Here's how the part is built. I have some questions about the finished solid (model axes, mm). Round coordinates to 2 decimals unless told otherwise and drop trailing zeros. Write each loop counter-clockwise with the first axis right and the second up, starting at its lowest first coordinate (ties: lowest second). Pieces come first, ordered by that corner, then holes. Notation, with made-up numbers: (35, 21) - (43, 21) arc R7 cw to (43, 30) - close; hole circle Ø7 at (-20.5, 4). An arc over 180 degrees is marked (long way). Use one line per item in the form item = value. Start each with the question number.
1. I want a section at B-B, the plane y = -19. List the corners of the cut face in (x, z) for me.
2. I want a section at A-A, the plane x = -59. List the corners of the cut face in (y, z) for me.
3. If I drill on line 1 along Y through (x, z) = (-31.5, -9.25); line 2 along Z through (x, y) = (-53, -25.5); line 3 along Y through (x, z) = (-32, 1.25), over which ranges is the centre line in solid material (lowest first)?
4. I want a section at C-C, the plane z = -15.75. List the corners of the cut face in (x, y) for me.
5. Will these pins go through, and if not, where does the flat tip stop? pin 1 (12 mm diameter, centred on x = -41.5, z = -4.5, fed in from +Y); pin 2 (3 mm diameter, centred on y = -25, z = -6.5, fed in from +X); pin 3 (1.8 mm diameter, centred on y = -25.5, z = -14, fed in from -X); pin 4 (6 mm diameter, centred on x = -67, y = -10, fed in from -Z).
```python
from build123d import *

# Parameters (mm, degrees)
CROQUIS1_W              = 50
CROQUIS1_H              = 50
CROQUIS1_R              = 1.5
SALIENTE_EXTRUIR1_DEPTH = 2
CROQUIS2_W              = 54
CROQUIS2_H              = 54
CROQUIS2_W_2            = 50
CROQUIS2_H_2            = 50
SALIENTE_EXTRUIR2_DEPTH = 2
CROQUIS3_W              = 2.1
CROQUIS3_H              = 6
SALIENTE_EXTRUIR3_DEPTH = 20


with BuildPart() as part:
    # Croquis1 → Saliente-Extruir1 (new body)
    with BuildSketch(Plane.XY):
        with Locations((-48.774779829, -1.232610977)):
            Rectangle(CROQUIS1_W, CROQUIS1_H)
        with Locations((-70.774779829, 20.767389023)):
            Circle(CROQUIS1_R, mode=Mode.SUBTRACT)
        with Locations((-26.774779829, 20.767389023)):
            Circle(CROQUIS1_R, mode=Mode.SUBTRACT)
        with Locations((-26.774779829, -23.232610977)):
            Circle(CROQUIS1_R, mode=Mode.SUBTRACT)
        with Locations((-70.774779829, -23.232610977)):
            Circle(CROQUIS1_R, mode=Mode.SUBTRACT)
        Polygon((-69.774779829, 17.767389023), (-67.774779829, 19.767389023), (-29.774779829, 19.767389023), (-27.774779829, 17.767389023), (-27.774779829, -20.232610977), (-29.774779829, -22.232610977), (-67.774779829, -22.232610977), (-69.774779829, -20.232610977), align=None, mode=Mode.SUBTRACT)
    extrude(amount=SALIENTE_EXTRUIR1_DEPTH)

    # Croquis2 → Saliente-Extruir2 (add)
    with BuildSketch(Plane(origin=(0, 0, 0), x_dir=(-1, 0, 0), z_dir=(0, 0, -1))):
        with Locations((48.774779829, -1.232610977)):
            Rectangle(CROQUIS2_W, CROQUIS2_H)
        with Locations((48.774779829, -1.232610977)):
            Rectangle(CROQUIS2_W_2, CROQUIS2_H_2, mode=Mode.SUBTRACT)
    extrude(amount=-SALIENTE_EXTRUIR2_DEPTH)

    # Croquis3 → Saliente-Extruir3 (add)
    with BuildSketch(Plane(origin=(0, 0, 0), x_dir=(-1, 0, 0), z_dir=(0, 0, -1))):
        with Locations((30.824779829, -25.232610977)):
            Rectangle(CROQUIS3_W, CROQUIS3_H)
    extrude(amount=SALIENTE_EXTRUIR3_DEPTH)


solid = part.part
```
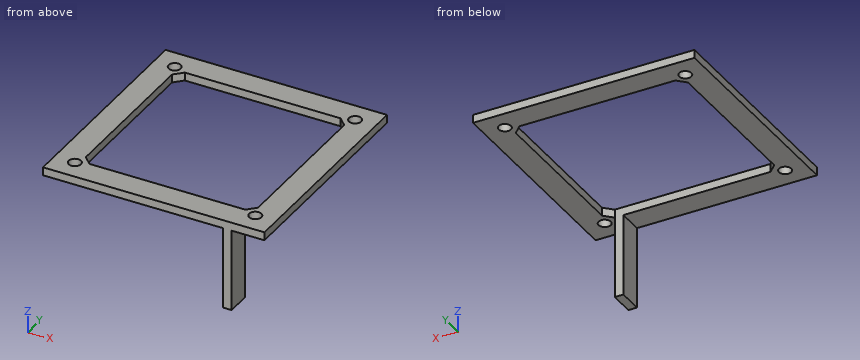
Model answer:
q1.outline = (-75.77, 0) - (-69.77, 0) - (-69.77, 2) - (-75.77, 2) - close; (-27.77, 0) - (-21.77, 0) - (-21.77, 2) - (-27.77, 2) - close
q2.outline = (-28.23, 0) - (-22.23, 0) - (-22.23, 2) - (-28.23, 2) - close; (19.77, 0) - (25.77, 0) - (25.77, 2) - (19.77, 2) - close
q3.line_1 = -28.23 to -22.23
q3.line_2 = 0 to 2
q3.line_3 = -28.23 to -22.23, 19.77 to 25.77
q4.outline = (-31.87, -28.23) - (-29.77, -28.23) - (-29.77, -22.23) - (-31.87, -22.23) - close
q5.pin_1 = 25.77
q5.pin_2 = -29.77
q5.pin_3 = -31.87
q5.pin_4 = 0
